Here's how the part is built. I have some questions about the finished solid (model axes, mm). A direction names the side the tool comes from. Coordinates: 2 decimals unless noted, no trailing zeros. Loops run counter-clockwise (first coordinate to the right, second up) from the corner with the lowest first, then second, coordinate; pieces in that order, holes last. Notation, with made-up numbers: (13, 25) -> (38, 25) arc R30 cw to (38, 57) -> close; hole circle Ø3 at (46, 16). An arc over 180 degrees is marked (long way). Answer as a JSON object with one key per item and string values. Group by question number.
1) I'm going to push flat-ended pins straight in: pin 1 (1.5 mm diameter, centred on x = 22, y = -21.5, fed in from -Z); pin 2 (2 mm diameter, centred on x = 15, z = 3.5, fed in from -Y); pin 3 (2 mm diameter, centred on x = -1.5, z = -7, fed in from -Y). Where does each tip first touch, or does it pass through?
2) I want a section at A-A (y = -24). Write out the boundary of the cut face in (x, z), then the cut area to 3 significant figures.
3) I want a section at C-C (x = 15). Write out the boundary of the cut face in (y, z).
4) Which directions (+Z, -Z, +X, -X, +Y, -Y) give clear straight access to the entire face, cutting with the end or side of a thin tool? Please do faces 1 (the flat face through (23.76, -23.4, 5.68)), 2 (the flat face through (19.24, -23.4, 3.12)), 3 (the flat face through (3.5, -1, -2)).
5) I need wall thicknesses on probe 1 along Z at (x, y) = (21.5, -15.5); probe 2 along X at (y, z) = (0.5, -8.5); probe 3 along Y at (x, z) = (10, 1). Which ranges of each line are inside material? Lowest first, please. Write a range as [from, to].
6) I want a section at B-B (z = -10.5). Write out the boundary of the cut face in (x, y), then the cut area to 3 significant figures.
```python
from build123d import *

# Parameters (mm, degrees)
F0_W     = 7
F0_H     = 7
F1_DEPTH = 16.51
F3_W     = 7
F3_H     = 7
F4_DEPTH = 19.5
F5_W     = 7
F5_H     = 7
F6_DEPTH = 22
F8_DEPTH = 15


with BuildPart() as f1:
    # F0 (on Top) → F1 (new body)
    with BuildSketch(Plane.XY):
        Rectangle(F0_W, F0_H)
    extrude(amount=-F1_DEPTH)

    # F3 (on face) → F4 (join, through all)
    with BuildSketch(Plane(origin=(0, 3.5, 0), x_dir=(-1, 0, 0), z_dir=(0, 1, 0))):
        with Locations((0, 3.5)):
            Rectangle(F3_W, F3_H)
    extrude(amount=-F4_DEPTH)

    # F5 (on face) → F6 (join, through all)
    with BuildSketch(Plane.YZ.offset(3.5)):
        with Locations((-12.5, 3.5)):
            Rectangle(F5_W, F5_H)
    extrude(amount=F6_DEPTH)

    # F7 (on face) → F8 (join)
    with BuildSketch(Plane.XZ.offset(16)):
        Polygon((23, 7), (20, 7), (18.5, 4.401924), (20, 1.803848), (23, 1.803848), (24.5, 4.401924), align=None)
    extrude(amount=F8_DEPTH)


solid = f1.part
```
Determined:
{
 "1": {"pin 1": "z = 1.8", "pin 2": "y = -16", "pin 3": "y = -3.5"},
 "2": {"outline": "(18.5, 4.4) -> (20, 1.8) -> (23, 1.8) -> (24.5, 4.4) -> (23, 7) -> (20, 7) -> close", "area": "23.4 mm^2"},
 "3": {"outline": "(-16, 0) -> (-9, 0) -> (-9, 7) -> (-16, 7) -> close"},
 "4": {"face 1": "+Z, +X, -Y", "face 2": "-Z, -X, -Y", "face 3": "+Z, -Z, +X, +Y"},
 "5": {"probe 1": "[0, 7]", "probe 2": "[-3.5, 3.5]", "probe 3": "[-16, -9]"},
 "6": {"outline": "(-3.5, -3.5) -> (3.5, -3.5) -> (3.5, 3.5) -> (-3.5, 3.5) -> close", "area": "49.0 mm^2"}
}
